Part model, mm, in its own coordinate system. Face numbers are marked on the shaded views. A direction names the side the tool comes from. Coordinates: 2 decimals unless noted, no trailing zeros. Write each loop counter-clockwise with the first axis right and the second up, starting at its lowest first coordinate (ties: lowest second). Pieces come first, ordered by that corner, then holes. Notation, with made-up numbers: (67, 26) -> (94, 26) arc R8 ccw to (94, 35) -> close; hole circle Ø1 at (13, -30.5). An arc over 180 degrees is marked (long way). Write item = value, one per line.
from build123d import *

# Parameters (mm, degrees)
SKETCH2_W                                       = 31.623
SKETCH2_H                                       = 47.371
SKETCH2_W_2                                     = 30.48
SKETCH2_H_2                                     = 46.355
BOSS_EXTRUDE1_DEPTH                             = 2.032
SKETCH3_W                                       = 35.2425
SKETCH3_H                                       = 50.8
SKETCH3_W_2                                     = 30.48
SKETCH3_H_2                                     = 46.355
BOSS_EXTRUDE2_DEPTH                             = 3.81
SKETCH4_W                                       = 35.2425
SKETCH4_H                                       = 50.8
BOSS_EXTRUDE3_DEPTH                             = 2.032
CUT_EXTRUDE1_REACH                              = 62.138
CUT_EXTRUDE2_REACH                              = 61.89
SKETCH6_W                                       = 1.778
SKETCH6_H                                       = 2.54
FILLET1_R                                       = 1.27
CSK_FOR_M3_FLAT_HEAD_MACHINE_SCREW1_D           = 3
CSK_FOR_M3_FLAT_HEAD_MACHINE_SCREW1_CSINK_D     = 5.4
CSK_FOR_M3_FLAT_HEAD_MACHINE_SCREW1_CSINK_ANGLE = 90


with BuildPart() as part:
    # Sketch2 → Boss-Extrude1 (new body)
    with BuildSketch(Plane.XY):
        with Locations((15.9385, 23.8125)):
            Rectangle(SKETCH2_W, SKETCH2_H)
        with Locations((15.875, 23.8125)):
            Rectangle(SKETCH2_W_2, SKETCH2_H_2, mode=Mode.SUBTRACT)
    extrude(amount=BOSS_EXTRUDE1_DEPTH)

    # Sketch3 → Boss-Extrude2 (add)
    with BuildSketch(Plane.XY.offset(2.032)):
        with Locations((15.71625, 23.8125)):
            Rectangle(SKETCH3_W, SKETCH3_H)
        with Locations((15.875, 23.8125)):
            Rectangle(SKETCH3_W_2, SKETCH3_H_2, mode=Mode.SUBTRACT)
    extrude(amount=BOSS_EXTRUDE2_DEPTH)

    # Sketch4 → Boss-Extrude3 (add)
    with BuildSketch(Plane.XY.offset(5.842)):
        with Locations((15.71625, 23.8125)):
            Rectangle(SKETCH4_W, SKETCH4_H)
    extrude(amount=BOSS_EXTRUDE3_DEPTH)

    # Sketch5 → Cut-Extrude1 (cut, up to next)
    with BuildSketch(Plane(origin=(31.75, 0, 0), x_dir=(0, 0, -1), z_dir=(1, 0, 0)), mode=Mode.PRIVATE) as cut_extrude1_sk1:
        with BuildLine():
            Line((1.27, 26.3525), (1.27, 21.2725))
            ThreePointArc((1.27, 21.2725), (0, 20.0025), (-1.27, 21.2725))
            Line((-1.27, 21.2725), (-1.27, 26.3525))
            ThreePointArc((-1.27, 26.3525), (0, 27.6225), (1.27, 26.3525))
        make_face()
    cut_extrude1_tool1 = extrude(cut_extrude1_sk1.sketch, amount=-CUT_EXTRUDE1_REACH, mode=Mode.PRIVATE) & part.part
    add(cut_extrude1_tool1.solids().sort_by_distance((31.75, 23.8125, 0))[0], mode=Mode.SUBTRACT)

    # Sketch6 → Cut-Extrude2 (cut, up to next)
    with BuildSketch(Plane.ZY.offset(-0.127), mode=Mode.PRIVATE) as cut_extrude2_sk1:
        with Locations((0.889, 45.72)):
            Rectangle(SKETCH6_W, SKETCH6_H)
    cut_extrude2_tool1 = extrude(cut_extrude2_sk1.sketch, amount=-CUT_EXTRUDE2_REACH, mode=Mode.PRIVATE) & part.part
    # Sketch6 → Cut-Extrude2 (cut, up to next)
    with BuildSketch(Plane.ZY.offset(-0.127), mode=Mode.PRIVATE) as cut_extrude2_sk2:
        with Locations((0.889, 1.905)):
            Rectangle(SKETCH6_W, SKETCH6_H)
    cut_extrude2_tool2 = extrude(cut_extrude2_sk2.sketch, amount=-CUT_EXTRUDE2_REACH, mode=Mode.PRIVATE) & part.part
    # Sketch6 → Cut-Extrude2 (cut, up to next)
    with BuildSketch(Plane.ZY.offset(-0.127), mode=Mode.PRIVATE) as cut_extrude2_sk3:
        with Locations((0.889, 23.8125)):
            Rectangle(SKETCH6_W, SKETCH6_H)
    cut_extrude2_tool3 = extrude(cut_extrude2_sk3.sketch, amount=-CUT_EXTRUDE2_REACH, mode=Mode.PRIVATE) & part.part
    add(cut_extrude2_tool1.solids().sort_by_distance((0.127, 45.72, 0.889))[0], mode=Mode.SUBTRACT)
    add(cut_extrude2_tool2.solids().sort_by_distance((0.127, 1.905, 0.889))[0], mode=Mode.SUBTRACT)
    add(cut_extrude2_tool3.solids().sort_by_distance((0.127, 23.8125, 0.889))[0], mode=Mode.SUBTRACT)

    # Fillet1
    fillet1_edges = [part.edges().sort_by_distance(p)[0] for p in [
        (0.381, 3.175, 1.778),
        (0.381, 0.635, 1.778),
        (0.381, 22.5425, 1.778),
        (0.381, 25.0825, 1.778),
        (0.381, 46.99, 1.778),
        (0.381, 44.45, 1.778),
    ]]
    fillet(fillet1_edges, radius=FILLET1_R - 0.0001)  # a hair under: the kernel refuses the full size

    # CSK for M3 Flat Head Machine Screw1 (through all)
    with Locations(Plane.XY.offset(7.874)):
        with Locations((15.875, 2.564617431), (15.875, 45.016869066)):
            CounterSinkHole(CSK_FOR_M3_FLAT_HEAD_MACHINE_SCREW1_D / 2, CSK_FOR_M3_FLAT_HEAD_MACHINE_SCREW1_CSINK_D / 2, counter_sink_angle=CSK_FOR_M3_FLAT_HEAD_MACHINE_SCREW1_CSINK_ANGLE)


solid = part.part
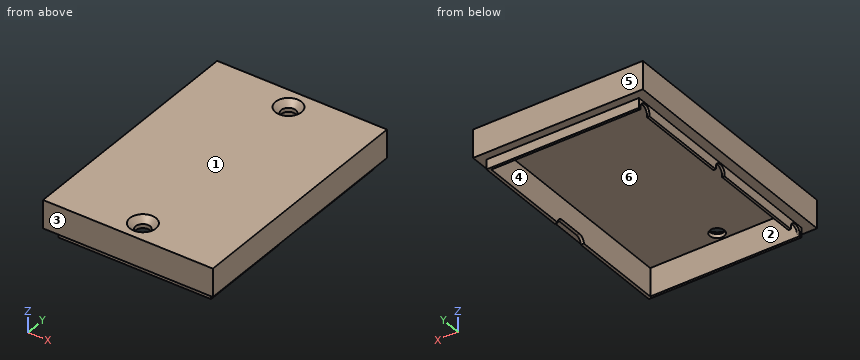
Q1. Mould opens along Y. For the marked faces 3, 4, 5 and 6 say: released by +Y, released by -Y, zero draft, split by the parting line, or undercut.
Model answer:
face_3 = released by -Y
face_4 = undercut
face_5 = released by +Y
face_6 = undercut
Q2. Saw through at A-A on x = 6. Give the cut face in (y, z) (1 decimal).
Model answer:
outline = (-1.6, 2) -> (0.1, 2) -> (0.1, 0) -> (0.6, 0) -> (0.6, 5.8) -> (47, 5.8) -> (47, 0) -> (47.5, 0) -> (47.5, 2) -> (49.2, 2) -> (49.2, 7.9) -> (-1.6, 7.9) -> close
Q3. Probe line 1 (X direction, y = 1.5, z = 4.25) (1 decimal); line 2 (Y direction, x = 26, z = 4) (1 decimal); line 3 (X direction, y = 44.5, z = 1) (3 decimals). List the from-to ranges inside material, lowest first. Write a range as from..to.
Model answer:
line_1 = -1.9..0.6, 31.1..33.3
line_2 = -1.6..0.6, 47..49.2
line_3 = 0.127..0.635, 31.115..31.75
Q4. Pin check, flat tips, straight feed: pin 1 (2 mm diameter, centred on x = 16, z = 1.5, fed in from +Y); pin 2 (2 mm diameter, centred on x = 20, z = 1, fed in from -Y); pin 3 (2 mm diameter, centred on y = 5, z = 1, fed in from -X); pin 4 (15 mm diameter, centred on x = 9.5, y = 19, fed in from -Z). Stop position of each tip, or through.
Model answer:
pin_1 = 49.21
pin_2 = 0.13
pin_3 = 0.13
pin_4 = 5.84
Q5. Saw through at B-B on z = 4.75. Give the cut face in (x, y) (1 decimal), and give its area (3 significant figures).
Model answer:
outline = (-1.9, -1.6) -> (33.3, -1.6) -> (33.3, 49.2) -> (-1.9, 49.2) -> close; hole (0.6, 0.6) -> (31.1, 0.6) -> (31.1, 47) -> (0.6, 47) -> close
area = 377 mm²
Q6. Which spindle directions (+Z, -Z, +X, -X, +Y, -Y) get a long thin tool onto all of the face, cutting with end or side? Do the marked faces 1 and 2. Say none if no direction does.
Model answer:
face_1 = +Z, +X, -X, +Y, -Y
face_2 = -Z
